Geometry check sheet. Reference: drawing and pictorial views, mm from the part's lowest x, y, z. Give positions to 0.01 mm unless a question says otherwise; leave off trailing zeros. Order: outer loops, then holes, each group sorted by start corner. A loop starts at its lowest first (then second) coordinate and runs counter-clockwise, first axis right, second up.
Item 1: Sectioned sample at D-D on y = 7.25. Record the boundary of the cut face in (x, z), and give its area (3 significant figures).
Item 2: Sectioned sample at B-B on x = 24.5. Record the boundary of the cut face in (y, z), and give its area (3 significant figures).
Item 3: Gauge pin test, flat end, axial feed: P1, Ø3, axis at x = 39, y = 7, coming from the +Z side. Record the tip position at first contact, or that the pin passes through.
Item 4: Material ranges on line 1 along Z through (x, y) = (24.5, 6.25); line 2 along Z through (x, y) = (39.5, 4.25), recorded low to high.
Item 5: Sectioned sample at A-A on z = 24.5. Record the boundary of the cut face in (x, y), and give its area (3 significant figures).
Item 6: Sectioned sample at C-C on y = 4.25. Record the boundary of the cut face in (x, z), and give its area (3 significant figures).
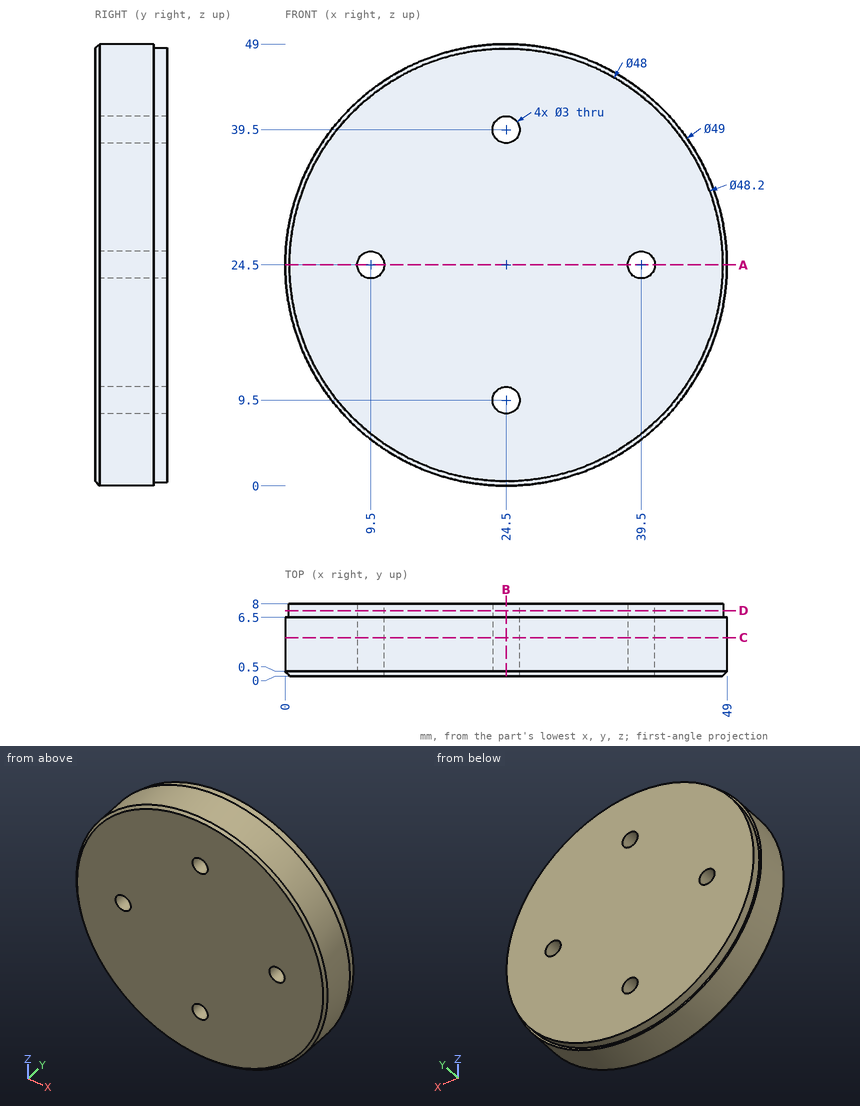
Report:
1. outline: circle Ø48.2 at (24.5, 24.5); hole circle Ø3 at (9.5, 24.5); hole circle Ø3 at (24.5, 9.5); hole circle Ø3 at (24.5, 39.5); hole circle Ø3 at (39.5, 24.5)
1. area: 1,800 mm2
2. outline: (0, 0.5) - (0.5, 0) - (6.5, 0) - (6.5, 0.4) - (8, 0.4) - (8, 8) - (0, 8) - close; (0, 11) - (8, 11) - (8, 38) - (0, 38) - close; (0, 41) - (8, 41) - (8, 48.6) - (6.5, 48.6) - (6.5, 49) - (0.5, 49) - (0, 48.5) - close
2. area: 343 mm2
3. P1: stops at z = 45.21
4. line 1: z = 0 to 8, 11 to 38, 41 to 49
4. line 2: z = 5.13 to 23, 26 to 43.87
5. outline: (0, 0.5) - (0.5, 0) - (8, 0) - (8, 8) - (0.4, 8) - (0.4, 6.5) - (0, 6.5) - close; (11, 0) - (38, 0) - (38, 8) - (11, 8) - close; (41, 0) - (48.5, 0) - (49, 0.5) - (49, 6.5) - (48.6, 6.5) - (48.6, 8) - (41, 8) - close
5. area: 343 mm2
6. outline: circle Ø49 at (24.5, 24.5); hole circle Ø3 at (9.5, 24.5); hole circle Ø3 at (24.5, 9.5); hole circle Ø3 at (24.5, 39.5); hole circle Ø3 at (39.5, 24.5)
6. area: 1,860 mm2
